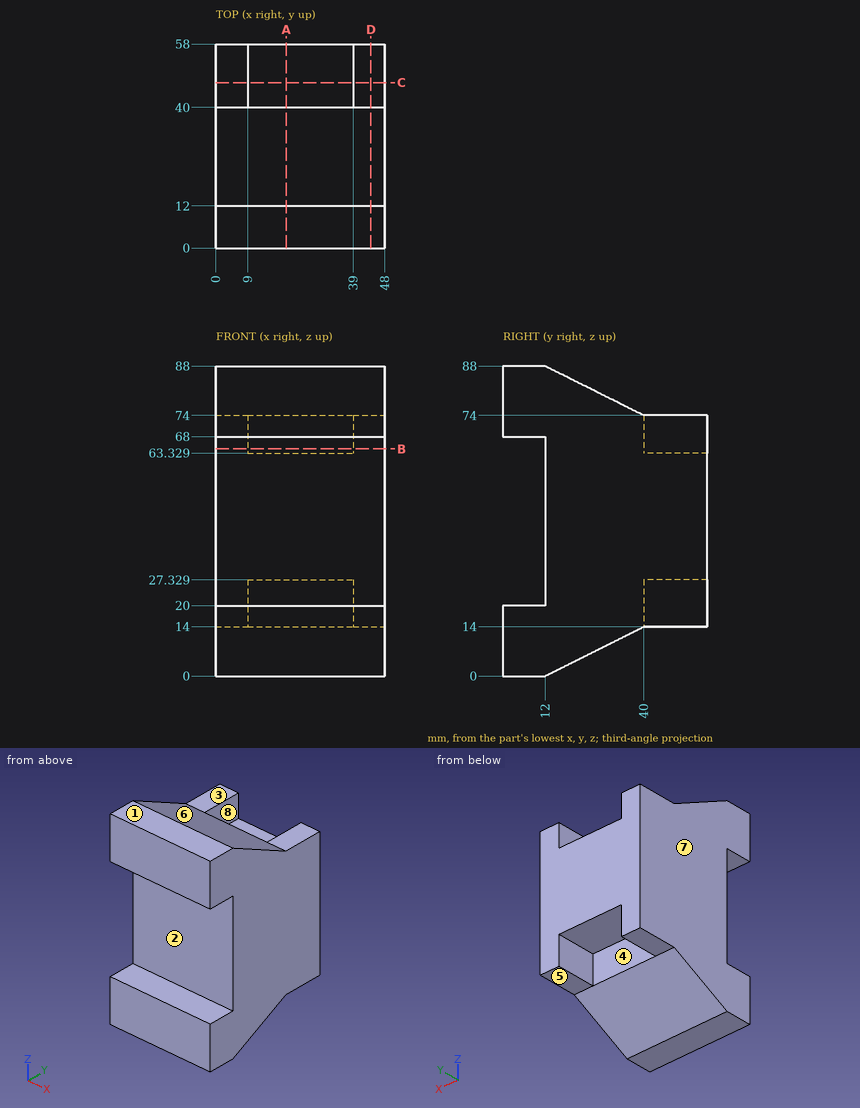
Verification items for this drawing (mm, ordinates from the low corner). A direction names the side the tool comes from. Give positions to 0.01 mm unless a question says otherwise; leave off trailing zeros. Loops run counter-clockwise (first coordinate to the right, second up) from the corner with the lowest first, then second, coordinate; pieces in that order, holes last. Notation, with made-up numbers: M 30.5,57.25 L 71.5,57.25 A27 ccw 71.5,74.25 Z; hole C 38,69 d5. An arc over 180 degrees is marked long. Answer as a JSON object with one key per item and string values. Group by question number.
Q1. Material ranges on line 1 along Z through (x, y) = (26, 46.5); line 2 along Y through (x, z) = (10, 37); line 3 along Z through (x, y) = (46, 44), recorded low to high. Write a range as [from, to].
Q2. Cross-section at B-B on z = 64.5. Record the cut outline in (x, y), then the cut area to 3 significant figures.
Q3. Access from +Z, -Z, +X, -X, +Y, -Y to the whole of each face (thin tool, end or side, straight path). Record for the marked faces 1, 2, 3, 4 and 5.
Q4. Cross-section at A-A on x = 20. Record the cut outline in (y, z).
Q5. Go/stop test with flat-tipped pins: P1, Ø6, axis at x = 33, z = 22, coming from the +Y side; P2, Ø10, axis at x = 6.5, y = 22.5, coming from the +Z side; P3, Ø5.5, axis at x = 26, y = 45, coming from the +Z side. Record where each tip stops, or that it passes through.
Q6. Cross-section at C-C on y = 47. Record the cut outline in (x, z).
Q7. Cross-section at D-D on x = 44. Record the cut outline in (y, z).
Q8. Release check for a two-part mould opening along X. For the marked faces 6, 7 and 8 record: released by +X, released by -X, zero draft, split by the parting line, or undercut.
Evaluation:
{
 "1": {"line 1": "z = [27.33, 63.33]", "line 2": "y = [12, 58]", "line 3": "z = [14, 74]"},
 "2": {"outline": "M 0,12 L 48,12 L 48,58 L 39,58 L 39,40 L 9,40 L 9,58 L 0,58 Z", "area": "1,670 mm2"},
 "3": {"face 1": "+Z, +X, -X, +Y, -Y", "face 2": "+X, -X, -Y", "face 3": "+Z, +X, -X, +Y", "face 4": "-Z, +Y", "face 5": "-Z, +X, -X, +Y"},
 "4": {"outline": "M 0,0 L 12,0 L 40,14 L 40,27.33 L 58,27.33 L 58,63.33 L 40,63.33 L 40,74 L 12,88 L 0,88 L 0,68 L 12,68 L 12,20 L 0,20 Z"},
 "5": {"P1": "stops at y = 40", "P2": "stops at z = 85.25", "P3": "stops at z = 63.33"},
 "6": {"outline": "M 0,14 L 9,14 L 9,27.33 L 39,27.33 L 39,14 L 48,14 L 48,74 L 39,74 L 39,63.33 L 9,63.33 L 9,74 L 0,74 Z"},
 "7": {"outline": "M 0,0 L 12,0 L 40,14 L 58,14 L 58,74 L 40,74 L 12,88 L 0,88 L 0,68 L 12,68 L 12,20 L 0,20 Z"},
 "8": {"face 6": "zero draft", "face 7": "released by -X", "face 8": "undercut"}
}
